from build123d import *

# Parameters (mm, degrees)
SKETCH1_W                                        = 222.25
SKETCH1_H                                        = 152.4
EXTRUDE1_DEPTH                                   = 25.4
SKETCH2_W                                        = 17.4625
SKETCH2_H                                        = 76.2
EXTRUDE2_DEPTH                                   = 117.475
SKETCH5_W                                        = 190.5
SKETCH5_H                                        = 152.4
CUT_EXTRUDE1_DEPTH                               = 0.79375
F_5_16_18_TAPPED_HOLE1_D                         = 6.5278
F_5_16_18_TAPPED_HOLE1_DEPTH                     = 22.9235
F_5_16_18_TAPPED_HOLE1_TIP                       = 1.961148974
F_5_16_18_TAPPED_HOLE2_D                         = 6.5278
F_5_16_18_TAPPED_HOLE2_DEPTH                     = 22.9235
F_5_16_18_TAPPED_HOLE2_TIP                       = 1.961148974
SKETCH9_R                                        = 4.7625
SKETCH9_R_2                                      = 3.175
EXTRUDE3_DEPTH                                   = 38.1
F_5_16_18_TAPPED_HOLE3_D                         = 6.5278
F_10_24_TAPPED_HOLE2_D                           = 3.7973
F_1_4_20_TAPPED_HOLE1_D                          = 5.1054
F_1_4_20_TAPPED_HOLE1_DEPTH                      = 16.51
F_1_4_20_TAPPED_HOLE1_TIP                        = 1.533816902
F_2_56_TAPPED_HOLE1_D                            = 1.778
F_2_56_TAPPED_HOLE1_DEPTH                        = 6.604
F_2_56_TAPPED_HOLE1_TIP                          = 0.53416509
F_10_24_TAPPED_HOLE3_D                           = 3.7973
F_10_24_TAPPED_HOLE3_DEPTH                       = 17.4625
SKETCH21_W                                       = 60.325
SKETCH21_H                                       = 12.7
CUT_EXTRUDE2_DEPTH                               = 6.35
FILLET1_R                                        = 9.525
CBORE_FOR_1_4_SOCKET_HEAD_CAP_SCREW1_D           = 6.5278
CBORE_FOR_1_4_SOCKET_HEAD_CAP_SCREW1_DEPTH       = 120.65
CBORE_FOR_1_4_SOCKET_HEAD_CAP_SCREW1_CBORE_D     = 11.1125
CBORE_FOR_1_4_SOCKET_HEAD_CAP_SCREW1_CBORE_DEPTH = 7.112


with BuildPart() as part:
    # Sketch1 → Extrude1 (new body)
    with BuildSketch(Plane(origin=(0, 0, 0), x_dir=(1, 0, 0), z_dir=(0, 1, 0))):
        Rectangle(SKETCH1_W, SKETCH1_H)
    extrude(amount=EXTRUDE1_DEPTH)

    # Sketch2 → Extrude2 (add)
    with BuildSketch(Plane(origin=(0, 3.175, 0), x_dir=(-1, 0, 0), z_dir=(0, 1, 0))):
        with Locations((119.85625, 0)):
            Rectangle(SKETCH2_W, SKETCH2_H)
        with Locations((-119.85625, 0)):
            Rectangle(SKETCH2_W, SKETCH2_H)
    extrude(amount=EXTRUDE2_DEPTH)

    # Sketch5 → Cut-Extrude1 (cut)
    with BuildSketch(Plane(origin=(0, 25.4, 0), x_dir=(-1, 0, 0), z_dir=(0, 1, 0))):
        Rectangle(SKETCH5_W, SKETCH5_H)
    extrude(amount=-CUT_EXTRUDE1_DEPTH, mode=Mode.SUBTRACT)

    # 5/16-18 Tapped Hole1
    with Locations(Plane(origin=(128.5875, 0, 0), x_dir=(0, 0, -1), z_dir=(1, 0, 0))):
        with Locations((-30.1625, 107.15625), (-30.1625, 18.25625), (30.1625, 18.25625), (30.1625, 107.15625)):
            Hole(F_5_16_18_TAPPED_HOLE1_D / 2, depth=F_5_16_18_TAPPED_HOLE1_DEPTH)
            with Locations((0, 0, -(F_5_16_18_TAPPED_HOLE1_DEPTH + F_5_16_18_TAPPED_HOLE1_TIP / 2))):  # 118° drill point
                Cone(0, F_5_16_18_TAPPED_HOLE1_D / 2, F_5_16_18_TAPPED_HOLE1_TIP, mode=Mode.SUBTRACT)

    # 5/16-18 Tapped Hole2
    with Locations(Plane.ZY.offset(128.5875)):
        with Locations((30.1625, 107.15625), (-30.1625, 107.15625), (-30.1625, 18.25625), (30.1625, 18.25625)):
            Hole(F_5_16_18_TAPPED_HOLE2_D / 2, depth=F_5_16_18_TAPPED_HOLE2_DEPTH)
            with Locations((0, 0, -(F_5_16_18_TAPPED_HOLE2_DEPTH + F_5_16_18_TAPPED_HOLE2_TIP / 2))):  # 118° drill point
                Cone(0, F_5_16_18_TAPPED_HOLE2_D / 2, F_5_16_18_TAPPED_HOLE2_TIP, mode=Mode.SUBTRACT)

    # Sketch9 → Extrude3 (add, symmetric)
    with BuildSketch(Plane.XY):
        with Locations((-111.125, 25.4)):
            Circle(SKETCH9_R)
        with Locations((-111.125, 3.175)):
            Circle(SKETCH9_R_2)
        with Locations((111.125, 3.175)):
            Circle(SKETCH9_R_2)
        with Locations((111.125, 25.4)):
            Circle(SKETCH9_R)
    extrude(amount=EXTRUDE3_DEPTH, both=True)

    # 5/16-18 Tapped Hole3 (through all)
    with Locations(Plane(origin=(0, 24.60625, 0), x_dir=(-1, 0, 0), z_dir=(0, 1, 0))):
        with Locations((0, 0), (50.8, -50.8), (50.8, 50.8), (-50.8, 50.8), (-50.8, -50.8), (76.2, 0), (-76.2, 0)):
            Hole(F_5_16_18_TAPPED_HOLE3_D / 2)

    # #10-24 Tapped Hole2 (through all)
    with Locations(Plane(origin=(0, 24.60625, 0), x_dir=(-1, 0, 0), z_dir=(0, 1, 0))):
        with Locations((38.1, 19.05), (38.1, -19.05), (0, -19.05), (0, 19.05), (-38.1, 19.05), (-38.1, -19.05)):
            Hole(F_10_24_TAPPED_HOLE2_D / 2)

    # 1/4-20 Tapped Hole1
    with Locations(Plane.ZY.offset(111.125)):
        with Locations((-68.2625, 12.7), (-68.2625, 20.6375)):
            Hole(F_1_4_20_TAPPED_HOLE1_D / 2, depth=F_1_4_20_TAPPED_HOLE1_DEPTH)
            with Locations((0, 0, -(F_1_4_20_TAPPED_HOLE1_DEPTH + F_1_4_20_TAPPED_HOLE1_TIP / 2))):  # 118° drill point
                Cone(0, F_1_4_20_TAPPED_HOLE1_D / 2, F_1_4_20_TAPPED_HOLE1_TIP, mode=Mode.SUBTRACT)

    # #2-56 Tapped Hole1
    with Locations(Plane(origin=(0, 24.60625, 0), x_dir=(-1, 0, 0), z_dir=(0, 1, 0))):
        with Locations((38.1, 0), (26.9875, 0), (-38.1, 0), (-26.9875, 0)):
            Hole(F_2_56_TAPPED_HOLE1_D / 2, depth=F_2_56_TAPPED_HOLE1_DEPTH)
            with Locations((0, 0, -(F_2_56_TAPPED_HOLE1_DEPTH + F_2_56_TAPPED_HOLE1_TIP / 2))):  # 118° drill point
                Cone(0, F_2_56_TAPPED_HOLE1_D / 2, F_2_56_TAPPED_HOLE1_TIP, mode=Mode.SUBTRACT)

    # #10-24 Tapped Hole3
    with Locations(Plane(origin=(128.5875, 0, 0), x_dir=(0, 0, -1), z_dir=(1, 0, 0))):
        with Locations((-4.7625, 114.3), (30.1625, 114.3)):
            Hole(F_10_24_TAPPED_HOLE3_D / 2, depth=F_10_24_TAPPED_HOLE3_DEPTH)

    # Sketch21 → Cut-Extrude2 (cut)
    with BuildSketch(Plane.ZY.offset(-111.125)):
        with Locations((-7.9375, 114.3)):
            Rectangle(SKETCH21_W, SKETCH21_H)
    extrude(amount=-CUT_EXTRUDE2_DEPTH, mode=Mode.SUBTRACT)

    # Fillet1
    # the kernel refuses this fillet: 9.525 mm, written as the material it adds along each edge
    with BuildSketch(Plane(origin=(117.475, 120.65, 22.225), x_dir=(0, 0, -1), z_dir=(0, -1, 0))) as fillet1_piece_1:
        with BuildLine():
            CenterArc((8.980256121, -9.525), FILLET1_R, 90, 70.528779366)
            Line((0, -6.35), (-0.179605122, -6.2865))
            ThreePointArc((-0.179605122, -6.2865), (-0.1905, -3.175), (-0.1905, 0))
            Line((-0.1905, 0), (0, 0.1905))
            Line((0, 0.1905), (8.980256121, 0.1905))
            Line((8.980256121, 0.1905), (8.980256121, 0))
        make_face()
    extrude(amount=35.150640303)

    # CBORE for 1/4 Socket Head Cap Screw1
    with Locations(Plane.XZ):
        with Locations((-50.8, 50.8), (50.8, 50.8), (50.8, -50.8), (0, 0), (-50.8, -50.8), (-76.2, 0), (76.2, 0)):
            CounterBoreHole(CBORE_FOR_1_4_SOCKET_HEAD_CAP_SCREW1_D / 2, CBORE_FOR_1_4_SOCKET_HEAD_CAP_SCREW1_CBORE_D / 2, CBORE_FOR_1_4_SOCKET_HEAD_CAP_SCREW1_CBORE_DEPTH, depth=CBORE_FOR_1_4_SOCKET_HEAD_CAP_SCREW1_DEPTH)


solid = part.part
Model file for the job. Use its own axes, mm. A direction names the side the tool comes from. Coordinates: 2 decimals unless noted, no trailing zeros. Loops run counter-clockwise (first coordinate to the right, second up) from the corner with the lowest first, then second, coordinate; pieces in that order, holes last. Notation, with made-up numbers: (31.5, 7) -> (58.5, 7) arc R23 cw to (58.5, 28) -> close; hole circle Ø9 at (-3.75, 24). An arc over 180 degrees is marked (long way). Use one line per item in the form item = value. Start each with the question number.
(1) Cut at D-D on z = -59. Give the cut face in (x, y) (3 decimals), and give its area (3 significant figures).
(2) Tool access for faces 1 (the conical face through (-93.348, 13.074, -68.024)), 2 (the flat face through (128.588, 61, -1)), 3 (the cylindrical face through (-56.35, 3.51, -50.56)), 4 (the flat face through (-111.125, 75, -1)), 5 (the flat face through (114, 107.95, -3)): list every direction of +Z, -Z, +X, -X, +Y, -Y with a clear straight run to the whole face (end or side of a thin tool).
(3) Pull direction Y, two halves, no side cores. Call faces 6 (the flat face through (1, 24.606, -16)), 7 (the cylindrical face through (-119.734, 109.908, -31.917)), 8 (the flat face through (-2, 0, 16)), 9 (the cylindrical face through (116.97, 15.07, -30.87)): pulls with the +Y half, pulls with the -Y half, needs draft (parallel to the pull), parting line crosses it, or undercut.
(4) Probe probe 1 along Z at (x, y) = (-50, 3); probe 2 along X at (y, z) = (32, 17) (1 decimal); probe 3 along Z at (x, y) = (-112, 57). List the from-to ranges inside material, lowest first. Write a range as from..to.
(5) Cut at B-B on y = 35. Give the cut face in (x, z) (1 decimal).
(6) Cut at C-C on x = -76.2. Give the cut face in (y, z).
(7) Flat gauge pins, fed straight in: pin 1 (5.5 mm diameter, centred on x = 48.5, z = 52.5, fed in from -Y); pin 2 (12.5 mm diameter, centred on y = 9, z = 66.5, fed in from -X) (3 decimals); pin 3 (2 mm diameter, centred on x = -50.5, z = -45.5, fed in from +Y); pin 4 (18 mm diameter, centred on x = 112, y = 88, fed in from +Z). Where does each tip first touch, or does it go through?
(8) Cut at A-A on x = 50.8. Give the cut face in (y, z).
Values:
q1.outline = (-111.125, 0) -> (111.125, 0) -> (111.125, 25.4) -> (95.25, 25.4) -> (95.25, 24.606) -> (-95.25, 24.606) -> (-95.25, 25.4) -> (-111.125, 25.4) -> close
q1.area = 5,490 mm2
q2.face_1 = -X
q2.face_2 = +Z, -Z, +X, +Y, -Y
q2.face_3 = -Y
q2.face_4 = +Z, -Z, +Y
q2.face_5 = -Z, +Y
q3.face_6 = pulls with the +Y half
q3.face_7 = undercut
q3.face_8 = pulls with the -Y half
q3.face_9 = undercut
q4.probe_1 = -76.2..-56.3, -45.3..45.3, 56.3..76.2
q4.probe_2 = -128.6..-111.1, 111.1..128.6
q4.probe_3 = -38.1..38.1
q5.outline = (-128.6, -38.1) -> (-111.1, -38.1) -> (-111.1, 38.1) -> (-128.6, 38.1) -> close; (111.1, -38.1) -> (128.6, -38.1) -> (128.6, 38.1) -> (111.1, 38.1) -> close
q6.outline = (0, -76.2) -> (24.61, -76.2) -> (24.61, -3.26) -> (7.11, -3.26) -> (7.11, -5.56) -> (0, -5.56) -> close; (0, 5.56) -> (7.11, 5.56) -> (7.11, 3.26) -> (24.61, 3.26) -> (24.61, 76.2) -> (0, 76.2) -> close
q7.pin_1 = 0
q7.pin_2 = -111.125
q7.pin_3 = 24.61
q7.pin_4 = 38.1
q8.outline = (0, -76.2) -> (24.61, -76.2) -> (24.61, -54.06) -> (7.11, -54.06) -> (7.11, -56.36) -> (0, -56.36) -> close; (0, -45.24) -> (7.11, -45.24) -> (7.11, -47.54) -> (24.61, -47.54) -> (24.61, 47.54) -> (7.11, 47.54) -> (7.11, 45.24) -> (0, 45.24) -> close; (0, 56.36) -> (7.11, 56.36) -> (7.11, 54.06) -> (24.61, 54.06) -> (24.61, 76.2) -> (0, 76.2) -> close
